Check sheet for the modelled part. Datum: model origin and axes. Units: mm. Face numbers are marked on the shaded views. A direction names the side the tool comes from. Coordinates: 2 decimals unless noted, no trailing zeros. Loops run counter-clockwise (first coordinate to the right, second up) from the corner with the lowest first, then second, coordinate; pieces in that order, holes last. Notation, with made-up numbers: (45, -4.5) - (54, -4.5) arc R16 ccw to (54, 22.5) - close; hole circle Ø2 at (20, -25.5). An arc over 180 degrees is marked (long way). Write each question's results on one line, items separated by ' | '. Start each with the question number.
1. Draft check along X on the marked faces 3, 4, 5 and 6. Enter one of: released by +X, released by -X, zero draft, split by the parting line, or undercut.
2. Cross-section at B-B (y = 23.5). Record the cut outline in (x, z), and give its area (3 significant figures).
3. Thickness scan on line 1 (X direction, y = 9.5, z = -11); line 2 (Z direction, x = -11, y = 25); line 3 (Y direction, x = -23.5, z = 13). Record the ranges inside material, lowest first. Write a range as [from, to].
4. Cross-section at A-A (z = -16). Record the cut outline in (x, y), and give its area (3 significant figures).
5. Gauge pin test, flat ends, axial feed: P1, Ø1.2, axis at x = 49, y = 13, coming from the -Z side; P2, Ø0.8, axis at x = 48, y = 13.5, coming from the +Z side; P3, Ø1.3, axis at y = 20.5, z = -18, coming from the +X side. Record the tip position at first contact, or that the pin passes through.
6. Tool access check on the marked faces 1 and 2. Record the directions out of +Z, -Z, +X, -X, +Y, -Y that give a thin tool (end or side, any length) a straight path to the whole face; none if there is none.
7. Cross-section at C-C (y = 15.5). Record the cut outline in (x, z), and give its area (3 significant figures).
8. Cross-section at D-D (x = -29). Record the cut outline in (y, z).
```python
from build123d import *

# Parameters (mm, degrees)
SKETCH1_W          = 100
SKETCH1_H          = 60
BASE_DEPTH         = 30
FILLET1_R          = 5
SHELL1_T           = -2.5
CUT_EXTRUDE1_REACH = 110.628
SKETCH2_W          = 20
SKETCH2_H          = 20
FILLET2_R          = 2.5
CUT_EXTRUDE2_REACH = 102.743
SKETCH4_W          = 20
SKETCH4_H          = 20
FILLET3_R          = 2.5
SKETCH5_W          = 5
SKETCH5_H          = 20
CUT_EXTRUDE3_DEPTH = 1
CUT_EXTRUDE5_REACH = 109.708
SKETCH8_W          = 5
SKETCH8_H          = 11


with BuildPart() as part:
    # Sketch1 → Base (new body)
    with BuildSketch(Plane(origin=(0, 0, 0), x_dir=(1, 0, 0), z_dir=(0, 1, 0))):
        Rectangle(SKETCH1_W, SKETCH1_H)
    extrude(amount=BASE_DEPTH)

    # Fillet1
    fillet1_edges = [part.edges().sort_by_distance(p)[0] for p in [
        (50, 15, 30),
        (-50, 15, 30),
        (-50, 15, -30),
        (50, 15, -30),
    ]]
    fillet(fillet1_edges, radius=FILLET1_R)

    # Shell1
    shell1_openings = [part.faces().sort_by_distance(p)[0] for p in [
        (0, 30, 0),
    ]]
    offset(amount=SHELL1_T, openings=shell1_openings, kind=Kind.INTERSECTION)

    # Sketch2 → Cut-Extrude1 (cut, up to next)
    with BuildSketch(Plane(origin=(50, 0, 0), x_dir=(0, 0, -1), z_dir=(1, 0, 0)), mode=Mode.PRIVATE) as cut_extrude1_sk1:
        with Locations((-10, 12.5)):
            Rectangle(SKETCH2_W, SKETCH2_H)
    cut_extrude1_tool1 = extrude(cut_extrude1_sk1.sketch, amount=-CUT_EXTRUDE1_REACH, mode=Mode.PRIVATE) & part.part
    add(cut_extrude1_tool1.solids().sort_by_distance((50, 12.5, 10))[0], mode=Mode.SUBTRACT)

    # Fillet2
    fillet2_edges = [part.edges().sort_by_distance(p)[0] for p in [
        (48.75, 2.5, 20),
        (48.75, 22.5, 20),
        (48.75, 22.5, 0),
        (48.75, 2.5, 0),
    ]]
    fillet(fillet2_edges, radius=FILLET2_R)

    # Sketch4 → Cut-Extrude2 (cut, up to next)
    with BuildSketch(Plane(origin=(-26.934652874, 4.896122142, -30), x_dir=(-1, 0, 0), z_dir=(0, 0, -1)), mode=Mode.PRIVATE) as cut_extrude2_sk1:
        with Locations((3.065347126, 7.603877858)):
            Rectangle(SKETCH4_W, SKETCH4_H)
    cut_extrude2_tool1 = extrude(cut_extrude2_sk1.sketch, amount=-CUT_EXTRUDE2_REACH, mode=Mode.PRIVATE) & part.part
    add(cut_extrude2_tool1.solids().sort_by_distance((-30, 12.5, -30))[0], mode=Mode.SUBTRACT)

    # Fillet3
    fillet3_edges = [part.edges().sort_by_distance(p)[0] for p in [
        (-20, 2.5, -28.75),
        (-20, 22.5, -28.75),
        (-40, 22.5, -28.75),
        (-40, 2.5, -28.75),
    ]]
    fillet(fillet3_edges, radius=FILLET3_R)

    # Sketch5 → Cut-Extrude3 (cut)
    with BuildSketch(Plane(origin=(50, 0, 0), x_dir=(0, 0, -1), z_dir=(1, 0, 0))):
        with Locations((17.5, 12.5)):
            Rectangle(SKETCH5_W, SKETCH5_H)
    extrude(amount=-CUT_EXTRUDE3_DEPTH, mode=Mode.SUBTRACT)

    # Sketch8 → Cut-Extrude5 (cut, up to next)
    with BuildSketch(Plane(origin=(49, 0, 0), x_dir=(0, 0, -1), z_dir=(1, 0, 0)), mode=Mode.PRIVATE) as cut_extrude5_sk1:
        with Locations((17.5, 12.5)):
            Rectangle(SKETCH8_W, SKETCH8_H)
    cut_extrude5_tool1 = extrude(cut_extrude5_sk1.sketch, amount=-CUT_EXTRUDE5_REACH, mode=Mode.PRIVATE) & part.part
    add(cut_extrude5_tool1.solids().sort_by_distance((49, 12.5, -17.5))[0], mode=Mode.SUBTRACT)


solid = part.part
```
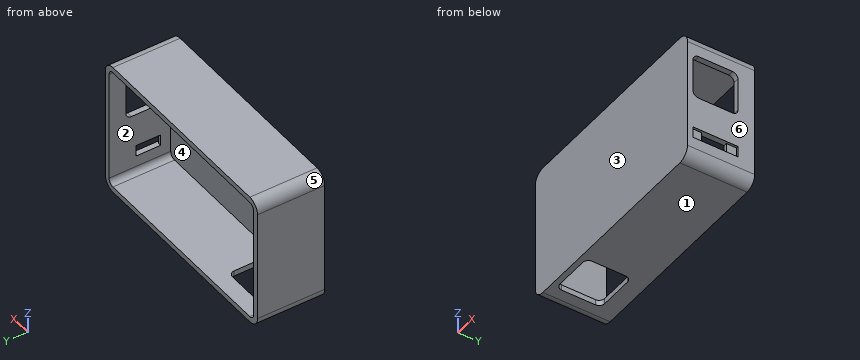
Established:
1) face 3: zero draft | face 4: undercut | face 5: released by -X | face 6: released by +X
2) outline: (-50, -25) arc R5 ccw to (-45, -30) - (45, -30) arc R5 ccw to (50, -25) - (50, 25) arc R5 ccw to (45, 30) - (-45, 30) arc R5 ccw to (-50, 25) - close; hole (-47.5, -25) arc R2.5 ccw to (-45, -27.5) - (45, -27.5) arc R2.5 ccw to (47.5, -25) - (47.5, 25) arc R2.5 ccw to (45, 27.5) - (-45, 27.5) arc R2.5 ccw to (-47.5, 25) - close | area: 759 mm^2
3) line 1: [-50, -47.5], [47.5, 50] | line 2: [-30, -27.5], [27.5, 30] | line 3: [0, 2.5]
4) outline: (-50, 0) - (50, 0) - (50, 2.5) - (49, 2.5) - (49, 7) - (47.5, 7) - (47.5, 2.5) - (-47.5, 2.5) - (-47.5, 30) - (-50, 30) - close; (47.5, 18) - (49, 18) - (49, 22.5) - (50, 22.5) - (50, 30) - (47.5, 30) - close | area: 351 mm^2
5) P1: z = -28.67 | P2: z = 29.27 | P3: x = 49
6) face 1: -Z, +X, -X, +Y, -Y | face 2: +Y
7) outline: (-50, -25) arc R5 ccw to (-45, -30) - (-40, -30) - (-40, -27.5) - (-45, -27.5) arc R2.5 cw to (-47.5, -25) - (-47.5, 25) arc R2.5 cw to (-45, 27.5) - (45, 27.5) arc R2.5 cw to (47.5, 25) - (47.5, 20) - (50, 20) - (50, 25) arc R5 ccw to (45, 30) - (-45, 30) arc R5 ccw to (-50, 25) - close; (-20, -30) - (45, -30) arc R5 ccw to (50, -25) - (50, -20) - (47.5, -20) - (47.5, -25) arc R2.5 cw to (45, -27.5) - (-20, -27.5) - close; (47.5, -15) - (50, -15) - (50, 0) - (47.5, 0) - close | area: 646 mm^2
8) outline: (0, -30) - (2.5, -30) - (2.5, 27.5) - (30, 27.5) - (30, 30) - (0, 30) - close; (22.5, -30) - (30, -30) - (30, -27.5) - (22.5, -27.5) - close
